from build123d import *

# Parameters (mm, degrees)
BOSS_EXTRUDE1_DEPTH = 3
BOSS_EXTRUDE2_DEPTH = 3


with BuildPart() as part:
    # Sketch2 → Boss-Extrude1 (new body)
    with BuildSketch(Plane.XY):
        Polygon((0, 0), (6, 1), (2, 5), (2, 3), (0, 1), align=None)
    extrude(amount=BOSS_EXTRUDE1_DEPTH)

    # Sketch3 → Boss-Extrude2 (add)
    with BuildSketch(Plane(origin=(0, 0, 0), x_dir=(-1, 0, 0), z_dir=(0, 0, -1))):
        Polygon((0, 0), (0, 1), (-4, 5), (-4, 3), (-6, 1), align=None)
    extrude(amount=BOSS_EXTRUDE2_DEPTH)


solid = part.part
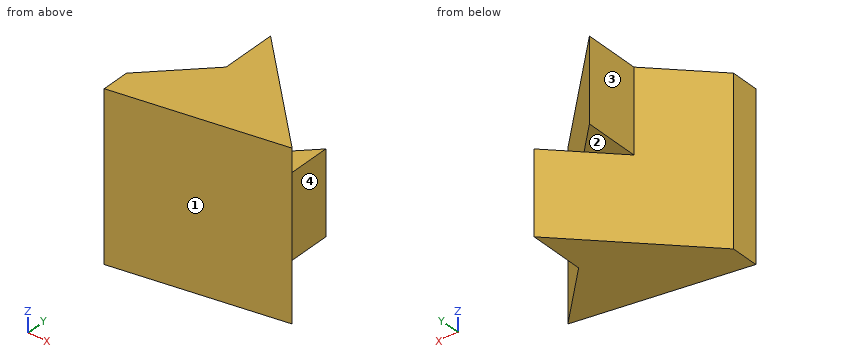
Part model, mm, in its own coordinate system. Face numbers are marked on the shaded views. A direction names the side the tool comes from. Coordinates: 2 decimals unless noted, no trailing zeros. Loops run counter-clockwise (first coordinate to the right, second up) from the corner with the lowest first, then second, coordinate; pieces in that order, holes last. Notation, with made-up numbers: M 70,72 L 119,72 A14 ccw 119,91 Z; hole C 10,-7 d11. An arc over 180 degrees is marked long. Use a Markdown table: item, result. Add a question column.
Q1. Probe L1, parallel to Z at x = 2.4, y = 3.8; L2, parallel to Z at x = 3.7, y = 4.2; L3, parallel to Y at x = 3.9, z = -1.5. List the from-to ranges inside material, lowest first.
Q2. Pin check, flat tips, straight feed: P1, Ø1.5, axis at y = 3.5, z = -1.5, coming from the +X side; P2, Ø0.8, axis at x = 3.5, y = 4, coming from the +Z side; P3, Ø1.6, axis at y = 3.5, z = -1, coming from the +X side; P4, Ø0.8, axis at x = 2.5, y = 4.5, coming from the -Z side. Stop position of each tip, or through.
Q3. Cut at C-C (z = -1.75). Write the cut outline in (x, y).
Q4. Cut at A-A (y = 4.1). Write the cut outline in (x, z).
Q5. Cut at D-D (y = 3.15). Write the cut outline in (x, z).
Q6. Which spindle directions (+Z, -Z, +X, -X, +Y, -Y) get a long thin tool onto all of the face, cutting with end or side? Do the marked faces 1, 2, 3 and 4. Say none if no direction does.
Q7. Cut at B-B (x = 3.6). Write the cut outline in (y, z).
Worked out:
| question | item | result |
|---|---|---|
| 1 | L1 | z = 0 to 3 |
| 1 | L2 | z = -3 to 0 |
| 1 | L3 | y = 0.65 to 4.9 |
| 2 | P1 | stops at x = 4.25 |
| 2 | P2 | stops at z = 3 |
| 2 | P3 | stops at x = 4.3 |
| 2 | P4 | stops at z = 0 |
| 3 | outline | M 0,0 L 6,1 L 4,3 L 4,5 L 0,1 Z |
| 4 | outline | M 2,0 L 2.9,0 L 2.9,3 L 2,3 Z; M 3.1,-3 L 4,-3 L 4,0 L 3.1,0 Z |
| 5 | outline | M 2,0 L 2.15,0 L 2.15,-3 L 4,-3 L 4,0 L 3.85,0 L 3.85,3 L 2,3 Z |
| 6 | face 1 | +Z, -Z, +X, -Y |
| 6 | face 2 | -Z, -X, +Y |
| 6 | face 3 | +Z, -Z, -X, +Y |
| 6 | face 4 | +Z, -Z, +X, +Y |
| 7 | outline | M 0.6,-3 L 4.6,-3 L 4.6,0 L 3.4,0 L 3.4,3 L 0.6,3 Z |
